Verification items for the finished model (mm, model axes). Round coordinates to 2 decimals unless told otherwise and drop trailing zeros. Loops run counter-clockwise (first coordinate to the right, second up) from the corner with the lowest first, then second, coordinate; pieces in that order, holes last. Notation, with made-up numbers: (63, 55.25) - (90, 55.25) arc R27 cw to (90, 82.25) - close; hole circle Ø10 at (44, -2). An arc over 180 degrees is marked (long way). Use CSV: the item, a comma, the result in double quotes.
```python
from build123d import *

# Parameters (mm, degrees)
F0_R     = 2.5
F0_R_2   = 1.01
F1_DEPTH = 25
F2_W     = 25
F2_H     = 10
F3_DEPTH = 1
F4_R     = 4.99999
F5_R     = 1


# Not quite as in the source:
# - a fillet or chamfer is up to 0.001 mm smaller than in the source, because OpenCascade refuses the exact size


with BuildPart() as f1:
    # F0 (on Top) → F1 (new body)
    with BuildSketch(Plane.XY):
        Circle(F0_R)
        Circle(F0_R_2, mode=Mode.SUBTRACT)
    extrude(amount=F1_DEPTH)

    # F2 (on Front) → F3 (join, symmetric)
    with BuildSketch(Plane.XZ):
        with Locations((0, 26.5656393021)):
            Rectangle(F2_W, F2_H)
    extrude(amount=F3_DEPTH, both=True)

    # F4 (radius 5 in the source; OpenCascade refuses exactly that, so slightly less here)
    f4_edges = [f1.edges().sort_by_distance(p)[0] for p in [
        (-12.5, 0, 21.565639),
        (-12.5, 0, 31.565639),
        (12.5, 0, 21.565639),
        (12.5, 0, 31.565639),
    ]]
    fillet(f4_edges, radius=F4_R)

    # F5
    f5_edges = [f1.edges().sort_by_distance(p)[0] for p in [
        (0, 2.5, 25),
        (0, -2.5, 25),
    ]]
    fillet(f5_edges, radius=F5_R)


solid = f1.part
```
1) Cross-section at A-A, the plane z = 24.5. Record the cut outline in (x, y), then the cut area to 3 significant figures.
Returned:
outline,"(-12.05, -1) - (-2.14, -1) arc R2.37 ccw to (2.14, -1) - (12.05, -1) - (12.05, 1) - (2.14, 1) arc R2.37 ccw to (-2.14, 1) - (-12.05, 1) - close; hole (-0.14, -1) arc R1.01 ccw to (0.14, -1) - close; hole (-0.14, 1) - (0.14, 1) arc R1.01 ccw to start"
area,"56.6 mm²"
2) Mould release check, pull along Y, two halves, no side actions. Record for faces 1 (the face through (-5, 0, 21.566)), 2 (the face through (-0.13, 1, 12.32)), 3 (the face through (-2.5, 0.1, 11.8)), 4 (the face through (0, 0, 21.566)): +Y half, -Y half, draft (parallel to the pull), parting line (faces both ways), or undercut.
Returned:
face 1,"draft"
face 2,"undercut"
face 3,"parting line"
face 4,"undercut"
3) Thickness scan on probe 1 along Y at (x, z) = (0, 12.5); probe 2 along Y at (x, z) = (10.25, 25.5); probe 3 along Z at (x, y) = (-6.5, -0.35). Record the ranges inside material, lowest first. Write a range as [from, to].
Returned:
probe 1,"y = [-2.5, -1.01], [1.01, 2.5]"
probe 2,"y = [-1, 1]"
probe 3,"z = [21.57, 31.57]"
4) Gauge pin test, flat ends, axial feed: pin 1 Ø2 at (y, z) = (-2, 19.5) entering from +X; pin 2 Ø5 at (x, z) = (0, 28) entering from +Y; pin 3 Ø3 at (x, z) = (3.5, 28.5) entering from -Y. Record the tip position at first contact, or that the pin passes through.
Returned:
pin 1,"stops at x = 2.29"
pin 2,"stops at y = 1"
pin 3,"stops at y = -1"
5) Cross-section at D-D, the plane x = -4.75. Record the cut outline in (y, z).
Returned:
outline,"(-1, 21.57) - (1, 21.57) - (1, 31.57) - (-1, 31.57) - close"
6) Cross-section at C-C, the plane z = 18.5. Record the cut outline in (x, y), then the cut area to 3 significant figures.
Returned:
outline,"circle Ø5 at (0, 0); hole circle Ø2.02 at (0, 0)"
area,"16.4 mm²"
